Geometry: final body of the model. Coordinates: model frame, mm. A direction names the side the tool comes from. Give positions to 0.01 mm unless a question says otherwise; leave off trailing zeros. Write each loop counter-clockwise with the first axis right and the second up, starting at its lowest first coordinate (ties: lowest second). Pieces come first, ordered by that corner, then holes.
Q1. Mould query, pull axis X, two halves, no side actions, for faces 1 (the cylindrical face through (11.923, 14.675, -3.755)), 2 (the flat face through (10, 29, -11)), 3 (the cylindrical face through (-25.865, 9.86, 10.724)). Classes: +X half, -X half, draft (parallel to the pull), parting line (faces both ways), or undercut.
Q2. Section C-C (y = 9.25). Return the cut outline in (x, z).
Q3. Section B-B (z = 0). Return the cut outline in (x, y).
Q4. Reachability of faces 4 (the flat face through (-25, 20, 6)), 5 (the flat face through (-12, 0, -12)) from +Z, -Z, +X, -X, +Y, -Y: full face, straight path, thin tool, end or side. Return the list, or none.
Q5. Section A-A (x = 0). Return the cut outline in (y, z).
Q6. Line query: line 1 (Z direction, x = 0, y = 14); line 2 (X direction, y = 8.25, z = 9); line 3 (Y direction, x = 25.5, z = 7.5). Output: solid intervals per line, ascending.
Q7. Pin query (flat end, axial travel): pin 1 Ø2 at (y, z) = (6.5, 5.5) entering from +X; pin 2 Ø1 at (x, y) = (-22, 6) entering from -Z; pin 3 Ø3 at (x, y) = (10.5, 15.5) entering from -Z. Return the tip coordinate at first contact, or that it passes through.
Autodesk Inventor part; units mm, degrees
ref_plane "YZ Plane" through (0, 0, 0) normal (1, 0, 0) x (0, 1, 0)
ref_plane "XZ Plane" through (0, 0, 0) normal (0, 1, 0) x (-1, 0, 0)
ref_plane "XY Plane" through (0, 0, 0) normal (0, 0, 1) x (1, 0, 0)
sketch "Sketch1" plane through (0, 0, 0) normal (0, 1, 0) x (-1, 0, 0)
  circle A0 centre (0, 0) radius 28
  dimension "d0" = 56
extrude "Extrusion1" add sketch "Sketch1" along normal blind 20
sketch "Sketch2" plane through (0, 20, 0) normal (0, 1, 0) x (1, 0, 0)
  circle A0 centre (0, 0) radius 23.5
  dimension "d3" = 47
extrude "Extrusion2" add sketch "Sketch2" along normal blind 9
sketch "Sketch3" plane through (0, 29, 0) normal (0, 1, 0) x (1, 0, 0)
  circle A0 centre (0, 0) radius 12.5
  dimension "d6" = 25
extrude "Extrusion3" cut sketch "Sketch3" against normal blind 38
fillet "Fillet1" radius 2 2 edges at (-12.5, 29, 0) (-12.5, 0, 0)
fillet "Fillet2" radius 2 1 edges at (-23.5, 20, 0)
properties part number "PISTON GUIDE"
Computed:
1. face 1: undercut
1. face 2: draft
1. face 3: parting line
2. outline: circle Ø56 at (0, 0); hole circle Ø25 at (0, 0)
3. outline: (-28, 0) - (-14.5, 0) arc R2 ccw to (-12.5, 2) - (-12.5, 27) arc R2 ccw to (-14.5, 29) - (-23.5, 29) - (-23.5, 22) arc R2 cw to (-25.5, 20) - (-28, 20) - close; (12.5, 2) arc R2 ccw to (14.5, 0) - (28, 0) - (28, 20) - (25.5, 20) arc R2 cw to (23.5, 22) - (23.5, 29) - (14.5, 29) arc R2 ccw to (12.5, 27) - close
4. face 4: +Y
4. face 5: +Z, -Z, +X, -X, -Y
5. outline: (0, -28) - (20, -28) - (20, -25.5) arc R2 cw to (22, -23.5) - (29, -23.5) - (29, -14.5) arc R2 ccw to (27, -12.5) - (2, -12.5) arc R2 ccw to (0, -14.5) - close; (0, 14.5) arc R2 ccw to (2, 12.5) - (27, 12.5) arc R2 ccw to (29, 14.5) - (29, 23.5) - (22, 23.5) arc R2 cw to (20, 25.5) - (20, 28) - (0, 28) - close
6. line 1: z = -28 to -12.5, 12.5 to 28
6. line 2: x = -26.51 to -8.67, 8.67 to 26.51
6. line 3: y = 0 to 20
7. pin 1: stops at x = 27.64
7. pin 2: stops at z = -17.94
7. pin 3: stops at z = -26.51
